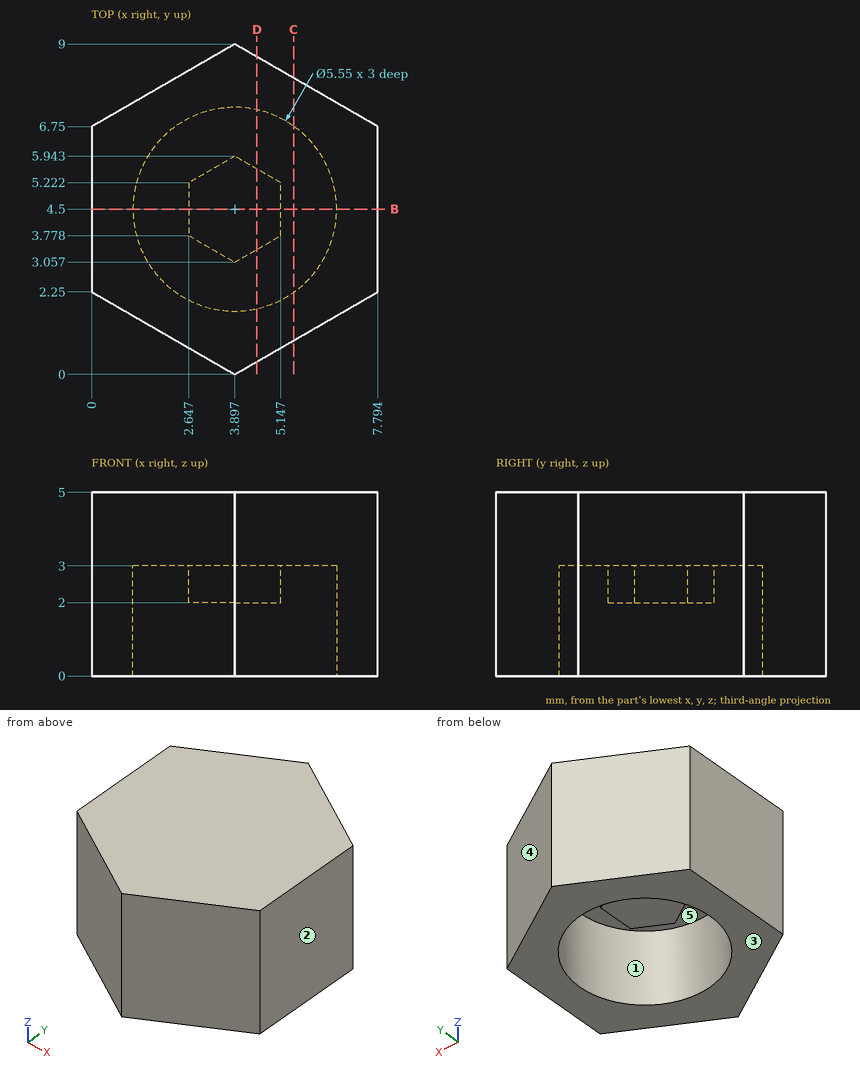
Part print with two shaded views. Sizes in mm from the minimum x, y, z corner. A direction names the side the tool comes from. Coordinates: 2 decimals unless noted, no trailing zeros. Order: outer loops, then holes, each group sorted by start corner. A loop starts at its lowest first (then second) coordinate and runs counter-clockwise, first axis right, second up. Notation, with made-up numbers: M -40,50.25 L -31,50.25 A20 cw -31,60.25 Z; hole C -13,50.25 d4. An arc over 180 degrees is marked long. One line per question, with ' | ' between items. Start each with the question number.
1. Cut at D-D (x = 4.5). Write the cut outline in (y, z) (1 decimal).
2. Mould opens along X. For the marked faces 3, 4 and 5 say: +X half, -X half, draft (parallel to the pull), parting line (faces both ways), or undercut.
3. Tool access for the marked faces 1 and 2: list every direction of +Z, -Z, +X, -X, +Y, -Y with a clear straight run to the whole face (end or side of a thin tool).
4. Cut at B-B (y = 4.5). Write the cut outline in (x, z), plus the area to 3 significant figures.
5. Cut at C-C (x = 5.5). Write the cut outline in (y, z) (1 decimal).
6. Flat gauge pin, fed straight in: P1, Ø0.8, axis at x = 4, y = 5, coming from the -Z side. Where does the tip first touch, or does it go through?
7. Wall check: line 1 along Y through (x, z) = (4.5, 2.3) (1 decimal); line 2 along Z through (x, y) = (3.25, 4); line 3 along Z through (x, y) = (3, 6). Give the ranges that are in metal, low to high. Write a range as [from, to].
The answers:
1) outline: M 0.3,0 L 1.8,0 L 1.8,3 L 3.4,3 L 3.4,2 L 5.6,2 L 5.6,3 L 7.2,3 L 7.2,0 L 8.7,0 L 8.7,5 L 0.3,5 Z
2) face 3: draft | face 4: +X half | face 5: undercut
3) face 1: -Z | face 2: +Z, -Z, +X, +Y, -Y
4) outline: M 0,0 L 1.12,0 L 1.12,3 L 2.65,3 L 2.65,2 L 5.15,2 L 5.15,3 L 6.67,3 L 6.67,0 L 7.79,0 L 7.79,5 L 0,5 Z | area: 24.8 mm2
5) outline: M 0.9,0 L 2.2,0 L 2.2,3 L 6.8,3 L 6.8,0 L 8.1,0 L 8.1,5 L 0.9,5 Z
6) P1: stops at z = 2
7) line 1: y = [0.3, 1.8], [3.4, 5.6], [7.2, 8.7] | line 2: z = [2, 5] | line 3: z = [3, 5]
